from build123d import *

# Parameters (mm, degrees)
F1_DEPTH = 5
F3_DEPTH = 5
F4_W     = 5
F4_H     = 25
F5_DEPTH = 20
F7_DEPTH = 25


with BuildPart() as f1:
    # F0 (on Top) → F1 (new body)
    with BuildSketch(Plane.XY):
        Polygon((0, 25), (0, 0), (12.5, 0), (12.5, -5), (20, -5), (20, 25), align=None)
    extrude(amount=F1_DEPTH)

    # F2 (on Right) → F3 (join)
    with BuildSketch(Plane.YZ):
        Polygon((10, 40), (0, 5), (25, 5), (25, 40), align=None)
    extrude(amount=F3_DEPTH)

    # F4 (on Right) → F5 (join)
    with BuildSketch(Plane.YZ):
        with Locations((12.5, 17.5)):
            Rectangle(F4_W, F4_H)
    extrude(amount=F5_DEPTH)

    # F6 (on Front) → F7 (cut)
    with BuildSketch(Plane.XZ):
        Polygon((20.343749, 30), (5, 30), (20.343749, 5), align=None)
    extrude(amount=-F7_DEPTH, mode=Mode.SUBTRACT)


solid = f1.part
Could you check a few things on this model? Use its own coordinates, in mm. A direction names the side the tool comes from. Coordinates: 2 decimals unless noted, no trailing zeros. Order: outer loops, then holes, each group sorted by start corner. A loop starts at its lowest first (then second) coordinate and runs counter-clockwise, first axis right, second up. Notation, with made-up numbers: (11.25, -36.5) -> (64.25, -36.5) arc R32 cw to (64.25, -4.5) -> close; hole circle Ø8 at (71, -1). An arc over 180 degrees is marked (long way). One line per question, with ' | ' between items.
Q1. Thinking about a two-plate mould opening in Z: for faces 1 (the face through (12, 20, 5)), 2 (the face through (6, 0, 2)), 3 (the face through (10, 10, 0)), which applies, pulls with the +Z half, pulls with the -Z half, needs draft (parallel to the pull), parting line crosses it, or undercut?
Return value:
face 1: pulls with the +Z half | face 2: needs draft | face 3: pulls with the -Z half
Q2. Imagine slicing it at B-B on z = 12.5. Please give me the cut outline in (x, y), and give its area (3 significant figures).
Return value:
outline: (0, 2.14) -> (5, 2.14) -> (5, 10) -> (15.74, 10) -> (15.74, 15) -> (5, 15) -> (5, 25) -> (0, 25) -> close | area: 168 mm²
Q3. Imagine slicing it at C-C on x = 2. Please give me the cut outline in (y, z).
Return value:
outline: (0, 0) -> (25, 0) -> (25, 40) -> (10, 40) -> (0, 5) -> close
Q4. Imagine slicing it at D-D on y = 5.5. Please give me the cut outline in (x, z).
Return value:
outline: (0, 0) -> (20, 0) -> (20, 5) -> (5, 5) -> (5, 24.25) -> (0, 24.25) -> close
Q5. I'm going to push flat-ended pins straight in: P1, Ø1.5, axis at y = 13.5, z = 33.5, coming from the +X side; P2, Ø1.5, axis at x = 6, z = 22, coming from the -Y side; P3, Ø7.5, axis at x = 13, z = 20.5, coming from the +Y side. Where does each tip first touch, or does it pass through?
Return value:
P1: x = 5 | P2: y = 10 | P3: y = 15
Q6. On a 3-axis mill with a long thin cutter (end or side, diameter ignored), from which of +Z, -Z, +X, -X, +Y, -Y can I reach the whole of each face in a straight line? I mean faces 4 (the face through (12, 4, 5)), 5 (the face through (5, 18, 23)), 6 (the face through (11, 15, 15)). Say none if no direction works.
Return value:
face 4: +Z, +X, -Y | face 5: +Z, +X | face 6: +Z, +X, +Y
Q7. If I drill on L1, parallel to X at y = 12.25, z = 31; L2, parallel to Y at x = 16.5, z = 9.5, over which ranges is the centre line in solid material (lowest first)?
Return value:
L1: 0 to 5 | L2: 10 to 15
Q8. Imagine slicing it at A-A on y = 12.75. Please give me the cut outline in (x, z).
Return value:
outline: (0, 0) -> (20, 0) -> (20, 5.56) -> (5, 30) -> (5, 40) -> (0, 40) -> close
